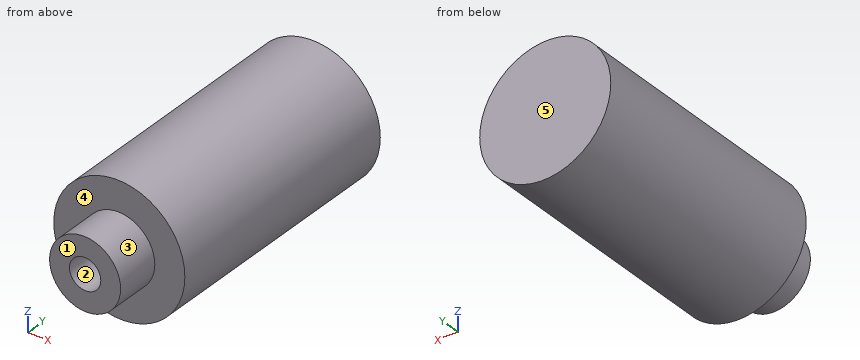
from build123d import *

# Parameters (mm, degrees)
CROQUIS1_R              = 10.25
SALIENTE_EXTRUIR1_DEPTH = 40
CROQUIS2_R              = 5.55
CROQUIS2_R_2            = 2.45
SALIENTE_EXTRUIR2_DEPTH = 7


with BuildPart() as part:
    # Croquis1 → Saliente-Extruir1 (new body)
    with BuildSketch(Plane(origin=(0, 0, 0), x_dir=(1, 0, 0), z_dir=(0, 1, 0))):
        Circle(CROQUIS1_R)
    extrude(amount=SALIENTE_EXTRUIR1_DEPTH)

    # Croquis2 → Saliente-Extruir2 (add)
    with BuildSketch(Plane.XZ):
        Circle(CROQUIS2_R)
        Circle(CROQUIS2_R_2, mode=Mode.SUBTRACT)
    extrude(amount=SALIENTE_EXTRUIR2_DEPTH)


solid = part.part
Can you work these out from the model? Positions are in its coordinate system, mm. Face numbers are marked on the shaded views. A direction names the side the tool comes from. Coordinates: 2 decimals unless noted, no trailing zeros. Write each loop counter-clockwise with the first axis right and the second up, starting at its lowest first coordinate (ties: lowest second). Pieces come first, ordered by that corner, then holes. Notation, with made-up numbers: (89.5, 73.5) - (118.5, 73.5) arc R30 ccw to (118.5, 101.5) - close; hole circle Ø5 at (41, 38.25). An arc over 180 degrees is marked (long way). Return JSON: item names as keys, results as strings. Group by question number.
Item 1: If we section it at A-A (z = 0): Write out the boundary of the cut face in (x, y).
Item 2: If we section it at D-D (z = -3): Write out the boundary of the cut face in (x, y).
Item 3: Please list where these lines run through material, in increasing order: probe 1 along Z at (x, y) = (0, -3); probe 2 along Y at (x, z) = (-2, 7.25); probe 3 along X at (y, z) = (29, -1).
Item 4: We'd pull the mould along Z, two halves only. Please class the marked faces 1, 2 and 3: pulls with the +Z half, pulls with the -Z half, needs draft (parallel to the pull), parting line crosses it, or undercut.
Item 5: If we section it at C-C (y = 12): Write out the boundary of the cut face in (x, z), then the cut area to 3 significant figures.
Item 6: If we section it at B-B (x = -2): Write out the boundary of the cut face in (y, z), then the cut area to 3 significant figures.
Item 7: Which directions (+Z, -Z, +X, -X, +Y, -Y) give clear straight access to the entire face, cutting with the end or side of a thin tool? Please do the marked faces 4 and 5.
Item 8: I'm going to push flat-ended pins straight in: pin 1 Ø1.5 at (x, z) = (0, -0.5) entering from -Y; pin 2 Ø10 at (x, y) = (5.5, 18.5) entering from +Z; pin 3 Ø1 at (y, z) = (1, 1.5) entering from -X. Where does each tip first touch, or does it pass through?
Return value:
{
 "1": {"outline": "(-10.25, 0) - (-5.55, 0) - (-5.55, -7) - (-2.45, -7) - (-2.45, 0) - (2.45, 0) - (2.45, -7) - (5.55, -7) - (5.55, 0) - (10.25, 0) - (10.25, 40) - (-10.25, 40) - close"},
 "2": {"outline": "(-9.8, 0) - (-4.67, 0) - (-4.67, -7) - (4.67, -7) - (4.67, 0) - (9.8, 0) - (9.8, 40) - (-9.8, 40) - close"},
 "3": {"probe 1": "z = -5.55 to -2.45, 2.45 to 5.55", "probe 2": "y = 0 to 40", "probe 3": "x = -10.2 to 10.2"},
 "4": {"face 1": "needs draft", "face 2": "undercut", "face 3": "parting line crosses it"},
 "5": {"outline": "circle Ø20.5 at (0, 0)", "area": "330 mm^2"},
 "6": {"outline": "(-7, -5.18) - (0, -5.18) - (0, -10.05) - (40, -10.05) - (40, 10.05) - (0, 10.05) - (0, 5.18) - (-7, 5.18) - (-7, 1.42) - (0, 1.42) - (0, -1.42) - (-7, -1.42) - close", "area": "857 mm^2"},
 "7": {"face 4": "-Y", "face 5": "+Z, -Z, +X, -X, +Y"},
 "8": {"pin 1": "stops at y = 0", "pin 2": "stops at z = 10.24", "pin 3": "stops at x = -10.2"}
}
